Design review of the part built by this model. Coordinates are the model's own, in mm. Face numbers are marked on the shaded views. A direction names the side the tool comes from. Coordinates: 2 decimals unless noted, no trailing zeros. Order: outer loops, then holes, each group sorted by start corner. A loop starts at its lowest first (then second) coordinate and runs counter-clockwise, first axis right, second up. Notation, with made-up numbers: M 42.25,58 L 52.25,58 A13 cw 52.25,76 Z; hole C -14.5,-35 d2. An arc over 180 degrees is marked long. Answer in a Markdown table with one row per item.
from build123d import *

# Parameters (mm, degrees)
F1_DEPTH = 101.6
F2_W     = 6.477
F2_H     = 1.5
F3_DEPTH = 19.5


with BuildPart() as f1:
    # F0 (on Front) → F1 (new body)
    with BuildSketch(Plane.XZ):
        Polygon((0, 14.34), (0, 0), (19.5, 0), (19.5, 14.34), (17.728965, 14.396643), (17.728965, 1.62), (1.548965, 1.62), (1.548965, 14.396643), align=None)
    extrude(amount=F1_DEPTH)

    # F2 (on face) → F3 (cut, through all)
    with BuildSketch(Plane(origin=(0, 0, 0), x_dir=(0, -1, 0), z_dir=(-1, 0, 0))):
        with Locations((7.9375, 0.75)):
            Rectangle(F2_W, F2_H)
        Polygon((90.551, 1.5), (90.551, 0), (96.901, 0), (97.028, 1.5), align=None)
    extrude(amount=-F3_DEPTH, mode=Mode.SUBTRACT)


solid = f1.part
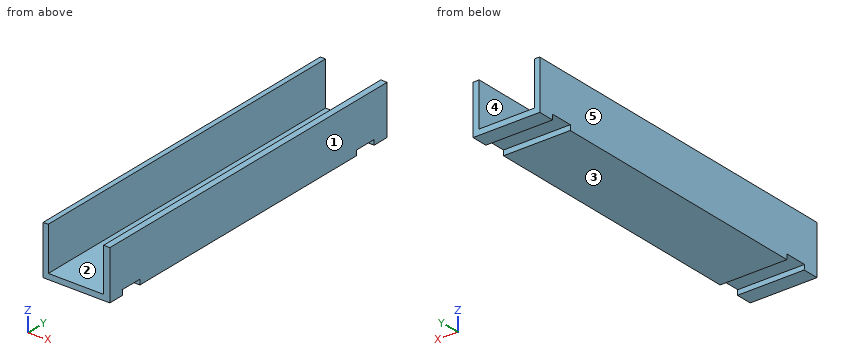
(1) Draft analysis for pull direction X (two halves, no side actions). For the marked faces 1, 2 and 3, state which applies: pulls with the +X half, pulls with the -X half, needs draft (parallel to the pull), parting line crosses it, or undercut.
Return value:
| item | result |
|---|---|
| face 1 | pulls with the +X half |
| face 2 | undercut |
| face 3 | needs draft |
(2) Add section C-C, the plane y = -65.5. Give the boundary of the cut face in (x, z), and give its area (3 significant figures).
Return value:
| item | result |
|---|---|
| outline | M 0,0 L 19.5,0 L 19.5,14.34 L 17.73,14.4 L 17.73,1.62 L 1.55,1.62 L 1.55,14.4 L 0,14.34 Z |
| area | 73.9 mm2 |
(3) For the marked faces 4 and 5, list the 3-axis set-ups (+Z, -Z, +X, -X, +Y, -Y) from which the entire face can be reached by the end or side of a thin tool; tool diameter is ignored.
Return value:
| item | result |
|---|---|
| face 4 | +Z, +Y, -Y |
| face 5 | +Z, -Z, -X, +Y, -Y |
(4) Add section A-A, the plane z = 11. Give the boundary of the cut face in (x, y).
Return value:
| item | result |
|---|---|
| outline | M 0,-101.6 L 1.55,-101.6 L 1.55,0 L 0,0 Z; M 17.73,-101.6 L 19.5,-101.6 L 19.5,0 L 17.73,0 Z |
(5) Insertion check: pin 1 Ø5 at (x, z) = (5.5, 6) entering from -Y; pin 2 Ø10 at (x, y) = (13, -85.5) entering from +Z; pin 3 Ø5 at (x, y) = (10.5, -93.5) entering from -Z; pin 4 Ø10 at (x, y) = (8.5, -80) entering from +Z. Each pin has a flat end and moves straight along its axis. Give the tip position at first contact, or say it passes through.
Return value:
| item | result |
|---|---|
| pin 1 | passes through |
| pin 2 | stops at z = 14.4 |
| pin 3 | stops at z = 1.5 |
| pin 4 | stops at z = 1.62 |
(6) Add section D-D, the plane y = -9. Give the boundary of the cut face in (x, z), and give its area (3 significant figures).
Return value:
| item | result |
|---|---|
| outline | M 0,1.5 L 19.5,1.5 L 19.5,14.34 L 17.73,14.4 L 17.73,1.62 L 1.55,1.62 L 1.55,14.4 L 0,14.34 Z |
| area | 44.7 mm2 |
(7) Add section B-B, the plane x = 11.5. Give the boundary of the cut face in (y, z), and give its area (3 significant figures).
Return value:
| item | result |
|---|---|
| outline | M -101.6,0 L -96.9,0 L -97.03,1.5 L -90.55,1.5 L -90.55,0 L -11.18,0 L -11.18,1.5 L -4.7,1.5 L -4.7,0 L 0,0 L 0,1.62 L -101.6,1.62 Z |
| area | 145 mm2 |
(8) For line 1 along Y through (x, z) = (7.75, 0.5); line 2 along X through (y, z) = (-63.5, 11); line 3 along Z through (x, y) = (18.25, -15), list the stretches that pass through material, from the lowest coordinate up. Write a range as from..to.
Return value:
| item | result |
|---|---|
| line 1 | y = -101.6..-96.94, -90.55..-11.18, -4.7..0 |
| line 2 | x = 0..1.55, 17.73..19.5 |
| line 3 | z = 0..14.38 |
